For this review, use the dimensioned drawing (mm, ordinates from the lowest corner) and the shaded views. Round coordinates to 2 decimals unless told otherwise and drop trailing zeros. Loops run counter-clockwise (first coordinate to the right, second up) from the corner with the lowest first, then second, coordinate; pieces in that order, holes last. Notation, with made-up numbers: (5.25, 33) - (14.25, 33) arc R34 cw to (14.25, 68) - close; hole circle Ø9 at (72.5, -20). An arc over 180 degrees is marked (long way). Return JSON: item names as keys, results as strings. Group by question number.
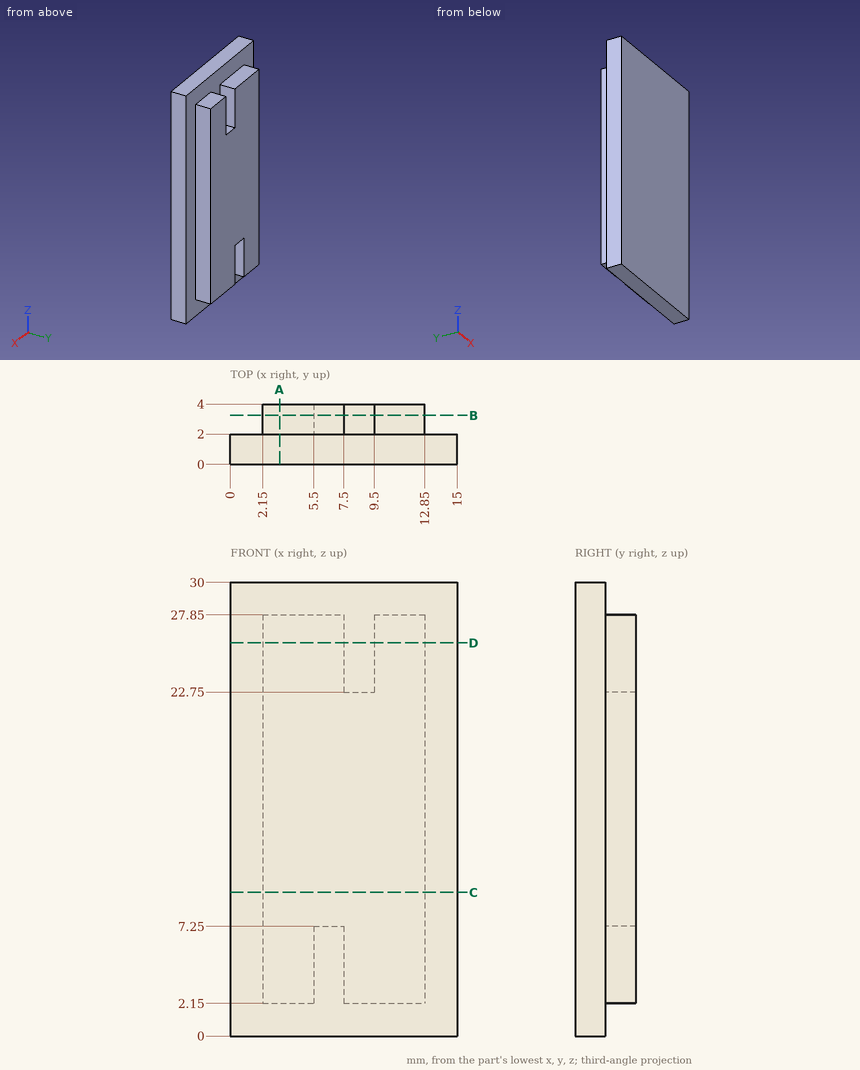
Q1. Insertion check: pin 1 Ø1.5 at (y, z) = (3, 8) entering from -X; pin 2 Ø0.6 at (x, y) = (10.5, 3.5) entering from +Z; pin 3 Ø1 at (y, z) = (3.5, 5) entering from +X. Each pin has a flat end and moves straight along its axis. Give the tip position at first contact, or say it passes through.
Q2. Add section B-B, the plane y = 3.25. State the section outline as (x, z) points.
Q3. Add section C-C, the plane z = 9.5. State the section outline as (x, y) points.
Q4. Add section D-D, the plane z = 26. State the section outline as (x, y) points, plus the area to 3 significant figures.
Q5. Add section A-A, the plane x = 3.25. State the section outline as (y, z) points.
Q6. For line 1 (X direction, y = 3.55, z = 3); line 2 (Y direction, x = 1.25, z = 3.75); line 3 (Z direction, x = 2.25, y = 2.6), list the stretches that pass through material, from the lowest coordinate up.
Evaluation:
{
 "1": {"pin 1": "x = 2.15", "pin 2": "z = 27.85", "pin 3": "x = 12.85"},
 "2": {"outline": "(2.15, 2.15) - (5.5, 2.15) - (5.5, 7.25) - (7.5, 7.25) - (7.5, 2.15) - (12.85, 2.15) - (12.85, 27.85) - (9.5, 27.85) - (9.5, 22.75) - (7.5, 22.75) - (7.5, 27.85) - (2.15, 27.85) - close"},
 "3": {"outline": "(0, 0) - (15, 0) - (15, 2) - (12.85, 2) - (12.85, 4) - (2.15, 4) - (2.15, 2) - (0, 2) - close"},
 "4": {"outline": "(0, 0) - (15, 0) - (15, 2) - (12.85, 2) - (12.85, 4) - (9.5, 4) - (9.5, 2) - (7.5, 2) - (7.5, 4) - (2.15, 4) - (2.15, 2) - (0, 2) - close", "area": "47.4 mm²"},
 "5": {"outline": "(0, 0) - (2, 0) - (2, 2.15) - (4, 2.15) - (4, 27.85) - (2, 27.85) - (2, 30) - (0, 30) - close"},
 "6": {"line 1": "2.15 to 5.5, 7.5 to 12.85", "line 2": "0 to 2", "line 3": "2.15 to 27.85"}
}
